```python
from build123d import *

# Parameters (mm, degrees)
F0_R     = 13
F0_R_2   = 5
F1_DEPTH = 8
F2_R     = 12
F2_R_2   = 11.5
F2_R_3   = 7
F2_R_4   = 6.5
F3_DEPTH = 1
F4_R     = 12
F4_R_2   = 11.5
F4_R_3   = 7
F4_R_4   = 6.5
F5_DEPTH = 1
F6_SIZE  = 0.5


with BuildPart() as f1:
    # F0 (on Front) → F1 (new body)
    with BuildSketch(Plane.XZ):
        Circle(F0_R)
        Circle(F0_R_2, mode=Mode.SUBTRACT)
    extrude(amount=F1_DEPTH)

    # F2 (on face) → F3 (cut)
    with BuildSketch(Plane.XZ.offset(8)):
        Circle(F2_R)
        Circle(F2_R_2, mode=Mode.SUBTRACT)
        Circle(F2_R_3)
        Circle(F2_R_4, mode=Mode.SUBTRACT)
    extrude(amount=-F3_DEPTH, mode=Mode.SUBTRACT)

    # F4 (on face) → F5 (cut)
    with BuildSketch(Plane(origin=(0, 0, 0), x_dir=(-1, 0, 0), z_dir=(0, 1, 0))):
        Circle(F4_R)
        Circle(F4_R_2, mode=Mode.SUBTRACT)
        Circle(F4_R_3)
        Circle(F4_R_4, mode=Mode.SUBTRACT)
    extrude(amount=-F5_DEPTH, mode=Mode.SUBTRACT)

    # F6
    f6_edges = [f1.edges().sort_by_distance(p)[0] for p in [
        (-13, 0, 0),
        (-5, 0, 0),
        (-5, -8, 0),
        (-13, -8, 0),
    ]]
    chamfer(f6_edges, length=F6_SIZE)


solid = f1.part
```
Model file for the job. Use its own axes, mm. A direction names the side the tool comes from. Give positions to 0.01 mm unless a question says otherwise; leave off trailing zeros. Order: outer loops, then holes, each group sorted by start corner. A loop starts at its lowest first (then second) coordinate and runs counter-clockwise, first axis right, second up.
1) Pin check, flat tips, straight feed: pin 1 (1.5 mm diameter, centred on x = -7, y = -5, fed in from +Z); pin 2 (3 mm diameter, centred on y = -4.5, z = -7.5, fed in from +X); pin 3 (1.5 mm diameter, centred on y = -7, z = -1, fed in from +X). Stop position of each tip, or through.
2) Wall check: probe 1 along Z at (x, y) = (0, -0.2); probe 2 along Z at (x, y) = (0, -7.45); probe 3 along Z at (x, y) = (0, -3.75). Give the ranges that are in metal, low to high.
3) 3-axis set-ups, long thin cutter, end or side, ignore diameter. For faces 1 (the flat face through (-7, 0, 10)), 2 (the cylindrical face through (-1.5, -7.5, 11.4)), 3 (the flat face through (-6, -1, -10)): which of +Z, -Z, +X, -X, +Y, -Y reach the whole face in a straight line?
4) Mould opens along Z. For faces 4 (the cylindrical face through (-10.316, -3.951, -7.91)), 5 (the cylindrical face through (-5.158, -7.507, -3.955)), 6 (the flat face through (-5, -8, 3)) say: +Z half, -Z half, draft (parallel to the pull), parting line (faces both ways), or undercut.
5) Saw through at A-A, the plane y = -4.75. Write the cut outline in (x, z).
Computed:
1. pin 1: stops at z = 11.4
1. pin 2: stops at x = 11.53
1. pin 3: stops at x = 13
2. probe 1: z = -12.7 to -12, -11.5 to -7, -6.5 to -5.3, 5.3 to 6.5, 7 to 11.5, 12 to 12.7
2. probe 2: z = -13 to -12, -11.5 to -7, -6.5 to -5, 5 to 6.5, 7 to 11.5, 12 to 13
2. probe 3: z = -13 to -5, 5 to 13
3. face 1: +Z, -Z, +X, -X, +Y
3. face 2: -Y
3. face 3: +Y
4. face 4: parting line
4. face 5: undercut
4. face 6: draft
5. outline: circle Ø26 at (0, 0); hole circle Ø10 at (0, 0)
